```python
from build123d import *

# Parameters (mm, degrees)
SKETCH_1_W          = 30
SKETCH_1_H          = 40
EXTRUDE_1_DEPTH     = 48
SHELL_1_T           = -3
SKETCH_2_R          = 1.75
CUT_EXTRUDE_1_DEPTH = 68.268120235
SKETCH_3_R          = 1.5
CUT_EXTRUDE_3_DEPTH = 70.310893805


with BuildPart() as part:
    # 草图1 → 凸台-拉伸1 (new body)
    with BuildSketch(Plane(origin=(0, 0, 0), x_dir=(1, 0, 0), z_dir=(0, 1, 0))):
        with Locations((15, -20)):
            Rectangle(SKETCH_1_W, SKETCH_1_H)
    extrude(amount=EXTRUDE_1_DEPTH)

    # 抽壳1
    shell_1_openings = [part.faces().sort_by_distance(p)[0] for p in [
        (15, 0, 20),
        (15, 24, 0),
        (30, 24, 20),
        (15, 24, 40),
    ]]
    offset(amount=SHELL_1_T, openings=shell_1_openings, kind=Kind.INTERSECTION)

    # 草图2 → 切除-拉伸1 (cut, through all)
    with BuildSketch(Plane.XZ.offset(-45)):
        with Locations(Location((11.5, 35, 0), (0, 0, 270))):
            Circle(SKETCH_2_R)
        with Locations(Location((21.5, 35, 0), (0, 0, 270))):
            Circle(SKETCH_2_R)
        with Locations(Location((21.5, 5, 0), (0, 0, 90))):
            Circle(SKETCH_2_R)
        with Locations(Location((11.5, 5, 0), (0, 0, 90))):
            Circle(SKETCH_2_R)
    extrude(amount=-CUT_EXTRUDE_1_DEPTH, mode=Mode.SUBTRACT)

    # 草图3 → 切除-拉伸3 (cut, through all)
    with BuildSketch(Plane.ZY):
        with Locations((27.75, 6.576606241)):
            Circle(SKETCH_3_R)
        with Locations((12.25, 6.576606241)):
            Circle(SKETCH_3_R)
        with Locations((4.5, 20)):
            Circle(SKETCH_3_R)
        with Locations((12.25, 33.423393759)):
            Circle(SKETCH_3_R)
        with Locations((27.75, 33.423393759)):
            Circle(SKETCH_3_R)
        with Locations((35.5, 20)):
            Circle(SKETCH_3_R)
        with BuildLine():
            Line((26.5, 20), (26.5, 29.252110748))
            ThreePointArc((26.5, 29.252110748), (20, 35.752110748), (13.5, 29.252110748))
            Line((13.5, 29.252110748), (13.5, 20))
            Line((13.5, 20), (13.5, 10.747889252))
            ThreePointArc((13.5, 10.747889252), (20, 4.247889252), (26.5, 10.747889252))
            Line((26.5, 10.747889252), (26.5, 20))
        make_face()
    extrude(amount=-CUT_EXTRUDE_3_DEPTH, mode=Mode.SUBTRACT)


solid = part.part
```
The model under review builds one solid part; all positions refer to its coordinate system, in mm. A direction names the side the tool comes from. Coordinates: 2 decimals unless noted, no trailing zeros. Write each loop counter-clockwise with the first axis right and the second up, starting at its lowest first coordinate (ties: lowest second). Pieces come first, ordered by that corner, then holes.
1) The part is to be moulded in two halves that separate along X. For faces 1 (the face through (0, 24, 29)), 2 (the face through (3, 22, 29)), 3 (the face through (23.235, 46.479, 35.228)), say which applies: pulls with the +X half, pulls with the -X half, needs draft (parallel to the pull), parting line crosses it, or undercut.
2) We need section A-A on z = 27.75. State the section outline as (x, y) points.
3) Clearance check with flat-ended pins moving along their axes: pin 1 Ø10 at (x, z) = (19.5, 30.5) entering from -Y; pin 2 Ø5 at (y, z) = (6.58, 12.25) entering from +X. State where each tip first meets the part, or that it passes through.
4) Machinability: for faces 4 (the face through (12.68, 46.48, 36.29)), 5 (the face through (16, 45, 20)), 6 (the face through (1, 20, 13.5)), which of the approach directions +Z, -Z, +X, -X, +Y, -Y give a long, thin tool a straight path to every point of the face, cutting with its end or side? Answer none if there is none.
5) We need section D-D on z = 20. State the section outline as (x, y) points, then the cut area to 3 significant figures.
6) We need section C-C on y = 13.5. State the section outline as (x, z) points, then the cut area to 3 significant figures.
7) To check wall thickness, follow probe 1 along X at (y, z) = (46, 35); probe 2 along Y at (x, z) = (1.8, 12.25); probe 3 along Y at (x, z) = (5, 29). State the ranges of each line that lie inside material, in increasing order.
8) We need section B-B on x = 11.5. State the section outline as (y, z) points, then the cut area to 3 significant figures.
Answer list:
1. face 1: pulls with the -X half
1. face 2: pulls with the +X half
1. face 3: undercut
2. outline: (0, 0) - (3, 0) - (3, 5.08) - (0, 5.08) - close; (0, 8.08) - (3, 8.08) - (3, 31.92) - (0, 31.92) - close; (0, 34.92) - (3, 34.92) - (3, 45) - (30, 45) - (30, 48) - (0, 48) - close
3. pin 1: stops at y = 45
3. pin 2: stops at x = 3
4. face 4: +Y, -Y
4. face 5: +Z, -Z, +X, -Y
4. face 6: +X, -X
5. outline: (0, 0) - (3, 0) - (3, 4.25) - (0, 4.25) - close; (0, 35.75) - (3, 35.75) - (3, 45) - (30, 45) - (30, 48) - (0, 48) - close
5. area: 130 mm2
6. outline: (0, 0) - (3, 0) - (3, 13.5) - (0, 13.5) - close; (0, 26.5) - (3, 26.5) - (3, 40) - (0, 40) - close
6. area: 81.0 mm2
7. probe 1: x = 0 to 9.75, 13.25 to 19.75, 23.25 to 30
7. probe 2: y = 0 to 5.08, 8.08 to 31.92, 34.92 to 48
7. probe 3: y = 45 to 48
8. outline: (45, 0) - (48, 0) - (48, 3.25) - (45, 3.25) - close; (45, 6.75) - (48, 6.75) - (48, 33.25) - (45, 33.25) - close; (45, 36.75) - (48, 36.75) - (48, 40) - (45, 40) - close
8. area: 99.0 mm2
